Could you check a few things on this model? Use its own coordinates, in mm. A direction names the side the tool comes from. Round coordinates to 2 decimals unless told otherwise and drop trailing zeros. Loops run counter-clockwise (first coordinate to the right, second up) from the corner with the lowest first, then second, coordinate; pieces in that order, holes last. Notation, with made-up numbers: (7.25, 6) -> (21.25, 6) arc R18 cw to (21.25, 16) -> close; hole circle Ø2 at (18.5, 25). An arc over 180 degrees is marked (long way). Write each question's results on one line, items separated by ' | '.
from build123d import *

# Parameters (mm, degrees)
SKETCH_1_W                         = 265
SKETCH_1_H                         = 186.75
SM_BASE_FLANGE_1_DEPTH             = 2
SM_EDGE_FLANGE_1_STRIP_W           = 9.4732
SM_EDGE_FLANGE_1_STRIP_H           = 2
SM_EDGE_FLANGE_1_STRIP_CUT_DEPTH   = 186.75
SM_EDGE_FLANGE_1_STRIP_2_W         = 9.4732
SM_EDGE_FLANGE_1_STRIP_2_H         = 2
SM_EDGE_FLANGE_1_STRIP_CUT_2_DEPTH = 186.75
SM_EDGE_FLANGE_1_DEPTH             = 186.75
SM_EDGE_FLANGE_1_BEND_DEPTH        = 186.75
SKETCH_12_R                        = 1.6
CUT_EXTRUDE_1_DEPTH                = 281


# Sheet-metal steps are written as plain solids
with BuildPart() as part:
    # Sketch 1 → Базовая кромка1 (new body)
    with BuildSketch(Plane(origin=(0, 0, 0), x_dir=(1, 0, 0), z_dir=(0, 1, 0))):
        with Locations((-90.995998399, -61.873281816)):
            Rectangle(SKETCH_1_W, SKETCH_1_H)
    extrude(amount=-SM_BASE_FLANGE_1_DEPTH)

    # Ребро-кромка1 strip (across the edge) → Ребро-кромка1 strip cut (cut)
    with BuildSketch(Plane(origin=(-223.495998399, 0, -31.501718184), x_dir=(1, 0, 0), z_dir=(0, 0, 1))):
        with Locations((-2, -1)):
            Rectangle(SM_EDGE_FLANGE_1_STRIP_W, SM_EDGE_FLANGE_1_STRIP_H)
    extrude(amount=SM_EDGE_FLANGE_1_STRIP_CUT_DEPTH, mode=Mode.SUBTRACT)

    # Ребро-кромка1 strip 2 (across the edge) → Ребро-кромка1 strip cut 2 (cut)
    with BuildSketch(Plane(origin=(41.504001601, 0, 155.248281816), x_dir=(-1, 0, 0), z_dir=(0, 0, -1))):
        with Locations((-2, -1)):
            Rectangle(SM_EDGE_FLANGE_1_STRIP_2_W, SM_EDGE_FLANGE_1_STRIP_2_H)
    extrude(amount=SM_EDGE_FLANGE_1_STRIP_CUT_2_DEPTH, mode=Mode.SUBTRACT)

    # Ребро-кромка1 section (across the edge) → Ребро-кромка1 (add)
    with BuildSketch(Plane(origin=(-223.495998399, 0, -31.501718184), x_dir=(1, 0, 0), z_dir=(0, 0, 1))):
        with BuildLine():
            Line((0, 0.7366), (0, 13))
            Line((0, 13), (2, 13))
            Line((2, 13), (2, 0.7366))
            ThreePointArc((2, 0.7366), (2.215745145, 0.215745145), (2.7366, 0))
            Line((2.7366, 0), (2.7366, -2))
            ThreePointArc((2.7366, -2), (0.801531583, -1.198468417), (0, 0.7366))
        make_face()
    extrude(amount=SM_EDGE_FLANGE_1_DEPTH)

    # Ребро-кромка1 section 2 (across the edge) → Ребро-кромка1 bend (add)
    with BuildSketch(Plane(origin=(41.504001601, 0, 155.248281816), x_dir=(-1, 0, 0), z_dir=(0, 0, -1))):
        with BuildLine():
            Line((0, 0.7366), (0, 13))
            Line((0, 13), (2, 13))
            Line((2, 13), (2, 0.7366))
            ThreePointArc((2, 0.7366), (2.215745145, 0.215745145), (2.7366, 0))
            Line((2.7366, 0), (2.7366, -2))
            ThreePointArc((2.7366, -2), (0.801531583, -1.198468417), (0, 0.7366))
        make_face()
    extrude(amount=SM_EDGE_FLANGE_1_BEND_DEPTH)

    # Эскиз12 → Вырез-Вытянуть1 (cut)
    with BuildSketch(Plane.ZY.offset(223.495998399)):
        with Locations(Location((-19.501718184, 8, 0), (0, 0, 270))):
            Circle(SKETCH_12_R)
        with Locations(Location((5.498281816, 8, 0), (0, 0, 270))):
            Circle(SKETCH_12_R)
    extrude(amount=-CUT_EXTRUDE_1_DEPTH, mode=Mode.SUBTRACT)


solid = part.part
1) If we mould it in two halves opening along X, with no side actions, what happens to faces 1 (the flat face through (39.504, 7, 63)), 2 (the flat face through (-223.496, 7, 61)), 3 (the flat face through (-93, 0, 61)), 4 (the flat face through (-92, -1, 155.248))? For each: released by +X, released by -X, zero draft, split by the parting line, or undercut.
Model answer:
face 1: undercut | face 2: released by -X | face 3: undercut | face 4: zero draft
2) I need wall thicknesses on line 1 (Z direction, x = 40.9, y = 8); line 2 (X direction, y = 1.25, z = -12.5); line 3 (Y direction, x = -70.5, z = -0.5). Which ranges of each line are inside material? Lowest first, please.
Model answer:
line 1: z = -31.5 to -21.1, -17.9 to 3.9, 7.1 to 155.25 | line 2: x = -223.5 to -221.5, 39.5 to 41.5 | line 3: y = -2 to 0
3) I want a section at A-A, the plane y = 3.5. Write out the boundary of the cut face in (x, z).
Model answer:
outline: (-223.5, -31.5) -> (-221.5, -31.5) -> (-221.5, 155.25) -> (-223.5, 155.25) -> close; (39.5, -31.5) -> (41.5, -31.5) -> (41.5, 155.25) -> (39.5, 155.25) -> close
4) For faces 5 (the flat face through (41.504, 7, 63)), 6 (the flat face through (-221.496, 7, 61)), which set-ups out of +Z, -Z, +X, -X, +Y, -Y let a thin tool reach every point of the face, with its end or its side?
Model answer:
face 5: +Z, -Z, +X, +Y, -Y | face 6: +Z, -Z, +Y
5) I want a section at B-B, the plane z = 70. Write out the boundary of the cut face in (x, y).
Model answer:
outline: (-223.5, 0.74) arc R2.74 ccw to (-220.76, -2) -> (38.77, -2) arc R2.74 ccw to (41.5, 0.74) -> (41.5, 13) -> (39.5, 13) -> (39.5, 0.74) arc R0.74 cw to (38.77, 0) -> (-220.76, 0) arc R0.74 cw to (-221.5, 0.74) -> (-221.5, 13) -> (-223.5, 13) -> close
6) I'm going to push a flat-ended pin straight in: pin 1 (1 mm diameter, centred on x = -70.5, z = 24, fed in from +Y). Where does the tip first touch, or does it pass through?
Model answer:
pin 1: stops at y = 0
7) I want a section at C-C, the plane x = -37. Write out the boundary of the cut face in (y, z), plus the area to 4 significant figures.
Model answer:
outline: (-2, -31.5) -> (0, -31.5) -> (0, 155.25) -> (-2, 155.25) -> close | area: 373.5 mm2
